Verification items for the finished model (mm, model axes). Round coordinates to 2 decimals unless told otherwise and drop trailing zeros. Write each loop counter-clockwise with the first axis right and the second up, starting at its lowest first coordinate (ties: lowest second). Pieces come first, ordered by that corner, then holes. Notation, with made-up numbers: M 39.5,33 L 62.5,33 A26 ccw 62.5,52 Z; hole C -16.5,-11 d1. An arc over 180 degrees is marked long. One line per item, written item: value. Start each with the question number.
Item 1: Section check D-D, the plane x = 38.3. Record the cut outline in (y, z), then the cut area to 3 significant figures.
Item 2: Section check C-C, the plane x = 27. Record the cut outline in (y, z), then the cut area to 3 significant figures.
Item 3: Thickness scan on probe 1 along Y at (x, z) = (27, 3.95); probe 2 along X at (y, z) = (19, 2.85); probe 3 along X at (y, z) = (50.5, 0.85). Record the ranges inside material, lowest first. Write a range as from..to.
Item 4: Section check B-B, the plane y = 42. Record the cut outline in (x, z), then the cut area to 3 significant figures.
Item 5: Section check A-A, the plane z = 4.85. Record the cut outline in (x, y).
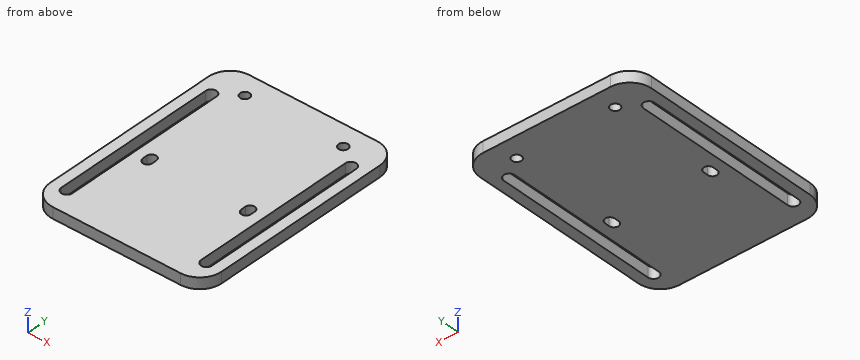
from build123d import *

# Parameters (mm, degrees)
MODEL_R    = 2.6
BASE_DEPTH = 6


with BuildPart() as part:
    # Model → Base (new body)
    with BuildSketch(Plane.XY):
        with BuildLine():
            Line((35, 0), (-35, 0))
            ThreePointArc((-35, 0), (-43.485281374, 3.514718626), (-47, 12))
            Line((-47, 12), (-47, 110.7))
            ThreePointArc((-47, 110.7), (-43.485281374, 119.185281374), (-35, 122.7))
            Line((-35, 122.7), (35, 122.7))
            ThreePointArc((35, 122.7), (43.485281374, 119.185281374), (47, 110.7))
            Line((47, 110.7), (47, 12))
            ThreePointArc((47, 12), (43.485281374, 3.514718626), (35, 0))
        make_face()
        with Locations((27, 110.7)):
            Circle(MODEL_R, mode=Mode.SUBTRACT)
        with Locations((-27, 110.7)):
            Circle(MODEL_R, mode=Mode.SUBTRACT)
        with BuildLine():
            Line((-29.6, 52.5), (-29.6, 50))
            ThreePointArc((-29.6, 50), (-27, 47.4), (-24.4, 50))
            Line((-24.4, 50), (-24.4, 52.5))
            ThreePointArc((-24.4, 52.5), (-27, 55.1), (-29.6, 52.5))
        make_face(mode=Mode.SUBTRACT)
        with BuildLine():
            Line((-41.3, 102.5), (-41.3, 12.5))
            ThreePointArc((-41.3, 12.5), (-38.3, 9.5), (-35.3, 12.5))
            Line((-35.3, 12.5), (-35.3, 102.5))
            ThreePointArc((-35.3, 102.5), (-38.3, 105.5), (-41.3, 102.5))
        make_face(mode=Mode.SUBTRACT)
        with BuildLine():
            Line((24.4, 52.5), (24.4, 50))
            ThreePointArc((24.4, 50), (27, 47.4), (29.6, 50))
            Line((29.6, 50), (29.6, 52.5))
            ThreePointArc((29.6, 52.5), (27, 55.1), (24.4, 52.5))
        make_face(mode=Mode.SUBTRACT)
        with BuildLine():
            Line((41.3, 12.5), (41.3, 102.5))
            ThreePointArc((41.3, 102.5), (38.3, 105.5), (35.3, 102.5))
            Line((35.3, 102.5), (35.3, 12.5))
            ThreePointArc((35.3, 12.5), (38.3, 9.5), (41.3, 12.5))
        make_face(mode=Mode.SUBTRACT)
    extrude(amount=BASE_DEPTH)


solid = part.part
Response values:
1. outline: M 0.46,0 L 9.5,0 L 9.5,6 L 0.46,6 Z; M 105.5,0 L 122.24,0 L 122.24,6 L 105.5,6 Z
1. area: 155 mm2
2. outline: M 0,0 L 47.4,0 L 47.4,6 L 0,6 Z; M 55.1,0 L 108.1,0 L 108.1,6 L 55.1,6 Z; M 113.3,0 L 122.7,0 L 122.7,6 L 113.3,6 Z
2. area: 659 mm2
3. probe 1: y = 0..47.4, 55.1..108.1, 113.3..122.7
3. probe 2: x = -47..-41.3, -35.3..35.3, 41.3..47
3. probe 3: x = -47..-41.3, -35.3..-29.6, -24.4..24.4, 29.6..35.3, 41.3..47
4. outline: M -47,0 L -41.3,0 L -41.3,6 L -47,6 Z; M -35.3,0 L 35.3,0 L 35.3,6 L -35.3,6 Z; M 41.3,0 L 47,0 L 47,6 L 41.3,6 Z
4. area: 492 mm2
5. outline: M -47,12 A12 ccw -35,0 L 35,0 A12 ccw 47,12 L 47,110.7 A12 ccw 35,122.7 L -35,122.7 A12 ccw -47,110.7 Z; hole M -41.3,12.5 A3 ccw -35.3,12.5 L -35.3,102.5 A3 ccw -41.3,102.5 Z; hole M -29.6,50 A2.6 ccw -24.4,50 L -24.4,52.5 A2.6 ccw -29.6,52.5 Z; hole C -27,110.7 d5.2; hole M 24.4,50 A2.6 ccw 29.6,50 L 29.6,52.5 A2.6 ccw 24.4,52.5 Z; hole C 27,110.7 d5.2; hole M 35.3,12.5 A3 ccw 41.3,12.5 L 41.3,102.5 A3 ccw 35.3,102.5 Z
